Read the model definition and answer for the solid it produces. Units are mm, in the model's axes. A direction names the side the tool comes from. Round coordinates to 2 decimals unless told otherwise and drop trailing zeros. Order: outer loops, then holes, each group sorted by start corner. A loop starts at its lowest first (then second) coordinate and runs counter-clockwise, first axis right, second up. Notation, with made-up numbers: (28, 49.5) -> (63, 49.5) arc R35 cw to (63, 86.5) -> close; hole circle Ø5 at (-33.5, 68). An arc over 180 degrees is marked (long way). Answer as a JSON object with one key per item and string values. Group by question number.
Item 1: Given P1, Ø2.5, axis at x = -3.5, y = 213.5, coming from the +Z side; P2, Ø5, axis at y = 214.5, z = 58, coming from the +X side; P3, Ø4, axis at x = 26, y = 230, coming from the +Z side; P4, Ø1.4, axis at y = 222.22, z = 69.89, coming from the +X side, each flat-ended and moving along its own axis, determine where each tip first touches the part or whether it passes through.
Item 2: Section C-C, the plane y = 218.75 is taken. Write down the section's boundary in (x, z), plus the area to 3 significant figures.
Item 3: Section B-B, the plane z = 66 is taken. Write down the section's boundary in (x, y).
Item 4: Consider probe 1 along X at (y, z) = (226.25, 59.25); probe 2 along Z at (x, y) = (-7, 226); probe 3 along Y at (x, z) = (21, 63). Determine where each line is inside the solid, lowest interval first. Write a range as from..to.
Item 5: Section A-A, the plane z = 60.25 is taken. Write down the section's boundary in (x, y).
Item 6: The mould has two halves that part along X. Classify faces 1 (the cylindrical face through (-10.77, 215.05, 63.63)), 2 (the flat face through (29.75, 222, 46)), 3 (the flat face through (20.25, 222, 61)): pulls with the +X half, pulls with the -X half, needs draft (parallel to the pull), parting line crosses it, or undercut.
Item 7: Section D-D, the plane x = -7.5 is taken. Write down the section's boundary in (y, z).
Item 8: For faces 4 (the flat face through (13, 217.223, 46)), 5 (the flat face through (-2, 231, 46.293)), 6 (the flat face through (13, 227.223, 46)), 7 (the flat face through (-9.25, 222, 61)), determine the directions among +Z, -Z, +X, -X, +Y, -Y from which every point of the face is accessible in a straight line to the end or side of a thin tool.
from build123d import *

# Parameters (mm, degrees)
SKETCH1_W                                        = 42
SKETCH1_H                                        = 22
BOSS_EXTRUDE1_DEPTH                              = 3
SKETCH2_W                                        = 13
SKETCH2_H                                        = 6
CUT_EXTRUDE1_DEPTH                               = 4
SKETCH3_W                                        = 13
SKETCH3_H                                        = 6
CUT_EXTRUDE2_DEPTH                               = 4
BOSS_EXTRUDE2_DEPTH                              = 3
BOSS_EXTRUDE3_DEPTH                              = 3
M2_CLEARANCE_HOLE1_D                             = 2.4
M2_CLEARANCE_HOLE1_CSINK_D                       = 2.45
M2_CLEARANCE_HOLE1_CSINK_ANGLE                   = 90
CBORE_FOR_M2_PAN_HEAD_MACHINE_SCREW1_D           = 2.4
CBORE_FOR_M2_PAN_HEAD_MACHINE_SCREW1_CBORE_D     = 5
CBORE_FOR_M2_PAN_HEAD_MACHINE_SCREW1_CBORE_DEPTH = 1.6


with BuildPart() as part:
    # Sketch1 → Boss-Extrude1 (new body)
    with BuildSketch(Plane.XY.offset(47.892560215)):
        with Locations((8.75, 222.222621224)):
            Rectangle(SKETCH1_W, SKETCH1_H)
    extrude(amount=-BOSS_EXTRUDE1_DEPTH)

    # Sketch2 → Cut-Extrude1 (cut, through all)
    with BuildSketch(Plane(origin=(0, 0, 44.892560215), x_dir=(-1, 0, 0), z_dir=(0, 0, -1))):
        with Locations((-13.146676675, 230.222621224)):
            Rectangle(SKETCH2_W, SKETCH2_H)
    extrude(amount=-CUT_EXTRUDE1_DEPTH, mode=Mode.SUBTRACT)

    # Sketch3 → Cut-Extrude2 (cut, through all)
    with BuildSketch(Plane(origin=(0, 0, 44.892560215), x_dir=(-1, 0, 0), z_dir=(0, 0, -1))):
        with Locations((-13.146676675, 214.222621224)):
            Rectangle(SKETCH3_W, SKETCH3_H)
    extrude(amount=-CUT_EXTRUDE2_DEPTH, mode=Mode.SUBTRACT)

    # Sketch4 → Boss-Extrude2 (add)
    with BuildSketch(Plane(origin=(-12.25, 0, 0), x_dir=(0, -1, 0), z_dir=(-1, 0, 0))):
        with BuildLine():
            Line((-231.222621224, 64.935707597), (-231.222621224, 47.892560215))
            Line((-231.222621224, 47.892560215), (-213.222621224, 47.892560215))
            Line((-213.222621224, 47.892560215), (-213.222621224, 64.839486293))
            ThreePointArc((-213.222621224, 64.839486293), (-222.179830351, 72.892432503), (-231.222621224, 64.935707597))
        make_face()
    extrude(amount=-BOSS_EXTRUDE2_DEPTH)

    # Sketch5 → Boss-Extrude3 (add)
    with BuildSketch(Plane(origin=(23.25, 0, 0), x_dir=(0, 0, -1), z_dir=(1, 0, 0))):
        with BuildLine():
            Line((-64.839486293, 213.222621224), (-47.892560215, 213.222621224))
            Line((-47.892560215, 213.222621224), (-47.892560215, 231.222621224))
            Line((-47.892560215, 231.222621224), (-64.935707597, 231.222621224))
            ThreePointArc((-64.935707597, 231.222621224), (-72.892432503, 222.179830351), (-64.839486293, 213.222621224))
        make_face()
    extrude(amount=-BOSS_EXTRUDE3_DEPTH)

    # M2 Clearance Hole1 (through all)
    with Locations(Plane(origin=(23.25, 0, 0), x_dir=(0, 0, -1), z_dir=(1, 0, 0))):
        with Locations((-63.892759177, 228.222223301), (-69.892560215, 222.222422263), (-63.892759177, 216.222621224), (-57.892958138, 222.222422263)):
            CounterSinkHole(M2_CLEARANCE_HOLE1_D / 2, M2_CLEARANCE_HOLE1_CSINK_D / 2, counter_sink_angle=M2_CLEARANCE_HOLE1_CSINK_ANGLE)

    # CBORE for M2 Pan Head Machine Screw1 (through all)
    with Locations(Plane.XY.offset(47.892560215)):
        with Locations((-3.353323325, 230.214980721), (-3.353323325, 214.214980721), (26.646676675, 214.214980721), (26.646676675, 230.214980721)):
            CounterBoreHole(CBORE_FOR_M2_PAN_HEAD_MACHINE_SCREW1_D / 2, CBORE_FOR_M2_PAN_HEAD_MACHINE_SCREW1_CBORE_D / 2, CBORE_FOR_M2_PAN_HEAD_MACHINE_SCREW1_CBORE_DEPTH)


solid = part.part
Values found:
{
 "1": {"P1": "z = 46.29", "P2": "x = 23.25", "P3": "z = 47.89", "P4": "through"},
 "2": {"outline": "(-12.25, 44.89) -> (29.75, 44.89) -> (29.75, 47.89) -> (23.25, 47.89) -> (23.25, 72.2) -> (20.25, 72.2) -> (20.25, 47.89) -> (-9.25, 47.89) -> (-9.25, 72.2) -> (-12.25, 72.2) -> close", "area": "272 mm2"},
 "3": {"outline": "(-12.25, 213.43) -> (-9.25, 213.43) -> (-9.25, 231.03) -> (-12.25, 231.03) -> close; (20.25, 213.43) -> (23.25, 213.43) -> (23.25, 231.03) -> (20.25, 231.03) -> close"},
 "4": {"probe 1": "-12.25..-9.25, 20.25..23.25", "probe 2": "44.89..47.89", "probe 3": "213.22..215.42, 217.02..227.42, 229.02..231.22"},
 "5": {"outline": "(-12.25, 213.22) -> (-9.25, 213.22) -> (-9.25, 231.22) -> (-12.25, 231.22) -> close; (20.25, 213.22) -> (23.25, 213.22) -> (23.25, 231.22) -> (20.25, 231.22) -> close"},
 "6": {"face 1": "needs draft", "face 2": "pulls with the +X half", "face 3": "undercut"},
 "7": {"outline": "(211.22, 44.89) -> (233.22, 44.89) -> (233.22, 47.89) -> (211.22, 47.89) -> close"},
 "8": {"face 4": "+Z, -Z, -Y", "face 5": "+Z", "face 6": "+Z, -Z, +Y", "face 7": "+Z, +Y, -Y"}
}
